The figure shows three views and two pictorial views of one solid part (mm, origin at its lowest corner). Answer the questions. A direction names the side the tool comes from. Coordinates: 2 decimals unless noted, no trailing zeros. Loops run counter-clockwise (first coordinate to the right, second up) from the corner with the lowest first, then second, coordinate; pieces in that order, holes last. Notation, with made-up numbers: (30.25, 85.25) -> (62.25, 85.25) arc R29 cw to (62.25, 114.25) -> close; hole circle Ø7 at (34, -12.5). An arc over 180 degrees is marked (long way). Answer in a Markdown table with one row per item.
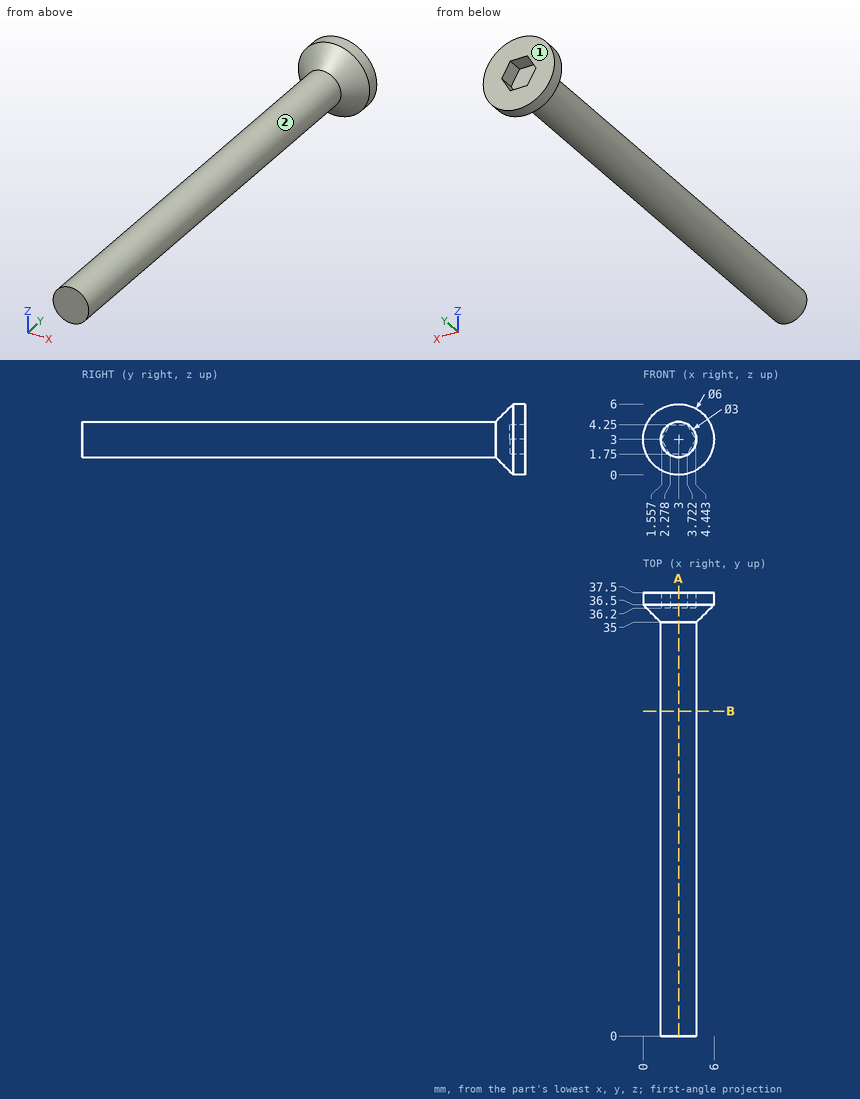
Item 1: A tool of negligible diameter and unlimited length cuts with its end or side. For the marked faces 1 and 2, from which of +Z, -Z, +X, -X, +Y, -Y can it reach the whole face along a straight path? Write none if from no direction.
Findings below:
| item | result |
|---|---|
| face 1 | +Z, -Z, +X, -X, +Y |
| face 2 | -Y |
Item 2: A cutting plane is placed at B-B, the plane y = 27.5. Determine the outline of the cut face in (x, z).
Findings below:
| item | result |
|---|---|
| outline | circle Ø3 at (3, 3) |
Item 3: Find the intervals of material crossed by probe 1 along Y at (x, z) = (2.9, 4); probe 2 along Z at (x, y) = (3.1, 32); probe 3 along Z at (x, y) = (2.1, 32.5), in increasing order.
Findings below:
| item | result |
|---|---|
| probe 1 | y = 0 to 36.2 |
| probe 2 | z = 1.5 to 4.5 |
| probe 3 | z = 1.8 to 4.2 |
Item 4: Flat-ended cylindrical pins translate along their axes: pin 1 Ø3 at (x, z) = (2.5, 3.5) entering from +Y; pin 2 Ø1.5 at (x, y) = (3, 22) entering from +Z; pin 3 Ø3 at (y, z) = (25, 1) entering from -X (1 decimal); pin 4 Ø2 at (x, y) = (1, 32) entering from +Z. Find the tip coordinate at first contact, or state that the pin passes through.
Findings below:
| item | result |
|---|---|
| pin 1 | stops at y = 37.5 |
| pin 2 | stops at z = 4.5 |
| pin 3 | stops at x = 1.6 |
| pin 4 | stops at z = 4.12 |
Item 5: A cutting plane is placed at A-A, the plane x = 3. Determine the outline of the cut face in (y, z).
Findings below:
| item | result |
|---|---|
| outline | (0, 1.5) -> (35, 1.5) -> (36.5, 0) -> (37.5, 0) -> (37.5, 1.75) -> (36.2, 1.75) -> (36.2, 4.25) -> (37.5, 4.25) -> (37.5, 6) -> (36.5, 6) -> (35, 4.5) -> (0, 4.5) -> close |
